Source: three-view drawing plus pictorial views. Frame: mm from the lowest corner of the part. A direction names the side the tool comes from. Give positions to 0.01 mm unless a question says otherwise; leave off trailing zeros. Write each loop counter-clockwise with the first axis right and the second up, starting at its lowest first coordinate (ties: lowest second). Pieces come first, ordered by that corner, then holes.
Q1. Cut plane D-D on y = 62. Return the cut outline in (x, z), plus the area to 3 significant figures.
Q2. Cut plane C-C on z = 4.5. Return the cut outline in (x, y).
Q3. Reachability of the marked faces 1 and 2 from +Z, -Z, +X, -X, +Y, -Y: full face, straight path, thin tool, end or side. Return the list, or none.
Q4. Pin query (flat end, axial travel): pin 1 (5 mm diameter, centred on y = 12.5, z = 24.5, fed in from -X); pin 2 (9 mm diameter, centred on x = 26.5, z = 19, fed in from -Y); pin 3 (2.5 mm diameter, centred on y = 9.34, z = 20.66, fed in from +X); pin 4 (2.5 mm diameter, centred on x = 12.5, y = 71, fed in from -Z). Return the tip coordinate at first contact, or that it passes through.
Q5. Line query: L1, parallel to X at y = 46, z = 17.5; L2, parallel to Y at x = 48.5, z = 3.75. Output: solid intervals per line, ascending.
Q6. Cut plane B-B on z = 23. Return the cut outline in (x, y).
Q7. Cut plane A-A on x = 10. Return the cut outline in (y, z), plus the area to 3 significant figures.
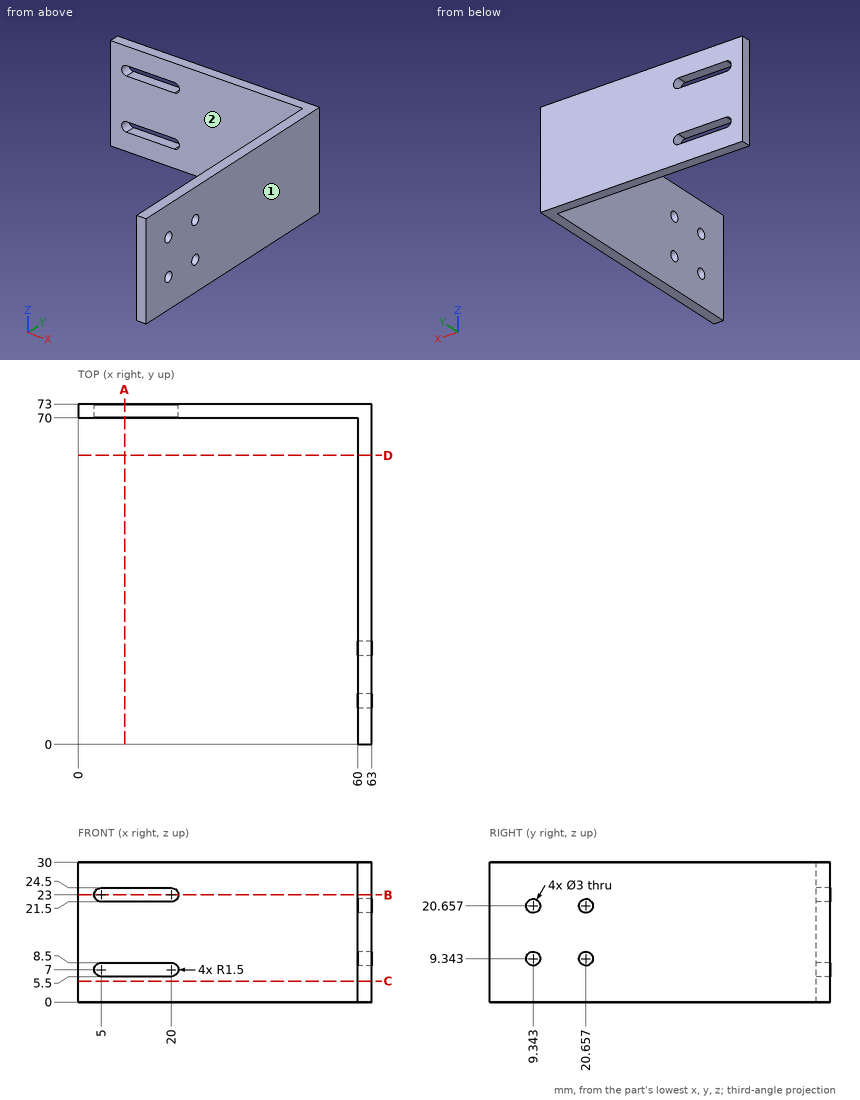
Data:
1. outline: (60, 0) - (63, 0) - (63, 30) - (60, 30) - close
1. area: 90.0 mm2
2. outline: (0, 70) - (60, 70) - (60, 0) - (63, 0) - (63, 73) - (0, 73) - close
3. face 1: +Z, -Z, +X, +Y, -Y
3. face 2: +Z, -Z, -X, -Y
4. pin 1: stops at x = 60
4. pin 2: stops at y = 70
4. pin 3: passes through
4. pin 4: stops at z = 0
5. L1: x = 60 to 63
5. L2: y = 70 to 73
6. outline: (0, 70) - (3.5, 70) - (3.5, 73) - (0, 73) - close; (21.5, 70) - (60, 70) - (60, 0) - (63, 0) - (63, 73) - (21.5, 73) - close
7. outline: (70, 0) - (73, 0) - (73, 5.5) - (70, 5.5) - close; (70, 8.5) - (73, 8.5) - (73, 21.5) - (70, 21.5) - close; (70, 24.5) - (73, 24.5) - (73, 30) - (70, 30) - close
7. area: 72.0 mm2
